```python
from build123d import *

# Parameters (mm, degrees)
SKETCH1_R           = 6.35
SKETCH1_R_2         = 1.5875
BOSS_EXTRUDE1_DEPTH = 6.35


with BuildPart() as part:
    # Sketch1 → Boss-Extrude1 (new body)
    # profile 1 of 3: a face of its own
    with BuildSketch(Plane.XY):
        with BuildLine():
            Line((33.528, 6.35), (0, 6.35))
            ThreePointArc((0, 6.35), (4.490128061, 4.490128061), (6.35, 0))
            ThreePointArc((6.35, 0), (4.490128061, -4.490128061), (0, -6.35))
            Line((0, -6.35), (33.528, -6.35))
            ThreePointArc((33.528, -6.35), (27.178, 0), (33.528, 6.35))
        make_face()
    # profile 2 of 3: a face of its own
    with BuildSketch(Plane.XY):
        Circle(SKETCH1_R)
        Circle(SKETCH1_R_2, mode=Mode.SUBTRACT)
    # profile 3 of 3: a face of its own
    with BuildSketch(Plane.XY):
        with Locations((33.528, 0)):
            Circle(SKETCH1_R)
        with Locations((33.528, 0)):
            Circle(SKETCH1_R_2, mode=Mode.SUBTRACT)
    extrude(amount=BOSS_EXTRUDE1_DEPTH)


solid = part.part
```
Input: part model. Units: mm. Frame: model coordinates. Give positions to 0.01 mm unless a question says otherwise; leave off trailing zeros. Order: outer loops, then holes, each group sorted by start corner. A loop starts at its lowest first (then second) coordinate and runs counter-clockwise, first axis right, second up.
1. Cut plane C-C (x = -1). Return loops of the section in (y, z), and give its area (3 significant figures).
Computed:
outline: (-6.27, 0) - (-1.23, 0) - (-1.23, 6.35) - (-6.27, 6.35) - close; (1.23, 0) - (6.27, 0) - (6.27, 6.35) - (1.23, 6.35) - close
area: 64.0 mm2
2. Draft query along Y for faces 1 (the face through (31.942, 0.07, 3.131)), 2 (the face through (-6.35, 0.14, 3.13)), 3 (the face through (17, -6.35, 3)), 4 (the face through (17, 6.35, 3)). Return one class per face: released by +Y, released by -Y, zero draft, split by the parting line, or undercut.
Computed:
face 1: undercut
face 2: split by the parting line
face 3: released by -Y
face 4: released by +Y
3. Pin query (flat end, axial travel): pin 1 Ø5 at (x, y) = (13, -1) entering from -Z. Return the tip coordinate at first contact, or that it passes through.
Computed:
pin 1: stops at z = 0
4. Cut plane A-A (y = 0). Return loops of the section in (x, z), and give its area (3 significant figures).
Computed:
outline: (-6.35, 0) - (-1.59, 0) - (-1.59, 6.35) - (-6.35, 6.35) - close; (1.59, 0) - (31.94, 0) - (31.94, 6.35) - (1.59, 6.35) - close; (35.12, 0) - (39.88, 0) - (39.88, 6.35) - (35.12, 6.35) - close
area: 253 mm2
5. Line query: probe 1 along X at (y, z) = (-0.5, 1); probe 2 along X at (y, z) = (1, 1.5); probe 3 along Y at (x, z) = (-1, 2.5). Output: solid intervals per line, ascending.
Computed:
probe 1: x = -6.33 to -1.51, 1.51 to 32.02, 35.03 to 39.86
probe 2: x = -6.27 to -1.23, 1.23 to 32.3, 34.76 to 39.8
probe 3: y = -6.27 to -1.23, 1.23 to 6.27
6. Cut plane D-D (y = 5.25). Return loops of the section in (x, z).
Computed:
outline: (-3.57, 0) - (37.1, 0) - (37.1, 6.35) - (-3.57, 6.35) - close
7. Cut plane B-B (z = 4.5). State how many separate pieces and enclosed holes the cut face has, and give its area (3 significant figures).
Computed:
separate pieces: 1
enclosed holes: 2
area: 537 mm2
